Could you check a few things on this model? Use its own coordinates, in mm. Coordinates: 2 decimals unless noted, no trailing zeros. Loops run counter-clockwise (first coordinate to the right, second up) from the corner with the lowest first, then second, coordinate; pieces in that order, holes last. Notation, with made-up numbers: M 37,86 L 44,86 A25 cw 44,112 Z; hole C 11.25,-3 d3. An arc over 180 degrees is marked long. Write each question's results on one line, items separated by ' | '.
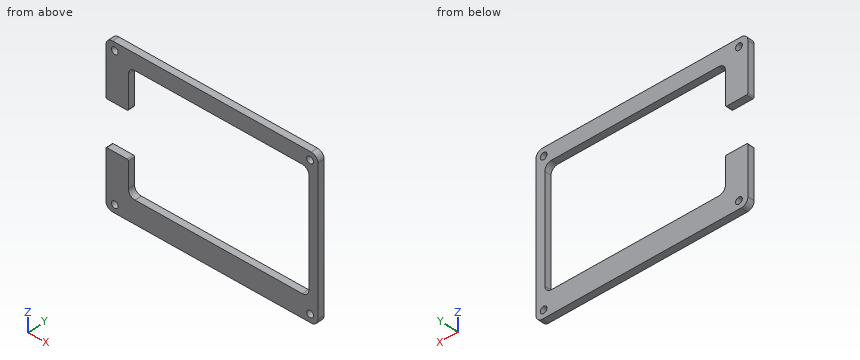
```python
from build123d import *

# Parameters (mm, degrees)
SKETCH1_W           = 94.5
SKETCH1_H           = 70
BOSS_EXTRUDE1_DEPTH = 3
SKETCH3_R           = 1.5
CUT_EXTRUDE2_DEPTH  = 59.877521177
FILLET2_R           = 3
SKETCH5_W           = 10
SKETCH5_H           = 20
CUT_EXTRUDE3_DEPTH  = 59.877521177
FILLET3_R           = 3
FILLET4_R           = 0.5


with BuildPart() as part:
    # Sketch1 → Boss-Extrude1 (new body)
    with BuildSketch(Plane(origin=(0, 0, 0), x_dir=(1, 0, 0), z_dir=(0, 1, 0))):
        Rectangle(SKETCH1_W, SKETCH1_H)
    extrude(amount=BOSS_EXTRUDE1_DEPTH)

    # Sketch3 → Cut-Extrude2 (cut, through all)
    with BuildSketch(Plane(origin=(0, 3, 0), x_dir=(1, 0, 0), z_dir=(0, 1, 0))):
        with Locations(Location((43.75, 31.5, 0), (0, 0, 270))):
            Circle(SKETCH3_R)
        with Locations(Location((-43.25, 31.5, 0), (0, 0, 270))):
            Circle(SKETCH3_R)
        with Locations(Location((-43.25, -31.5, 0), (0, 0, 270))):
            Circle(SKETCH3_R)
        with Locations(Location((43.75, -31.5, 0), (0, 0, 270))):
            Circle(SKETCH3_R)
    extrude(amount=-CUT_EXTRUDE2_DEPTH, mode=Mode.SUBTRACT)

    # Fillet2
    fillet2_edges = [part.edges().sort_by_distance(p)[0] for p in [
        (47.25, 1.5, 35),
        (-47.25, 1.5, 35),
        (-47.25, 1.5, -35),
        (47.25, 1.5, -35),
    ]]
    fillet(fillet2_edges, radius=FILLET2_R)

    # Sketch5 → Cut-Extrude3 (cut, through all)
    with BuildSketch(Plane(origin=(0, 3, 0), x_dir=(1, 0, 0), z_dir=(0, 1, 0))):
        Polygon((-30, -28), (-37.25, -28), (-37.25, 25), (43.25, 25), (43.25, -28), align=None)
        with Locations((-42.25, 0)):
            Rectangle(SKETCH5_W, SKETCH5_H)
    extrude(amount=-CUT_EXTRUDE3_DEPTH, mode=Mode.SUBTRACT)

    # Fillet3
    fillet3_edges = [part.edges().sort_by_distance(p)[0] for p in [
        (43.25, 1.5, 28),
        (-37.25, 1.5, 28),
        (-37.25, 1.5, -25),
        (43.25, 1.5, -25),
    ]]
    fillet(fillet3_edges, radius=FILLET3_R)

    # Fillet4
    fillet4_edges = [part.edges().sort_by_distance(p)[0] for p in [
        (-37.25, 1.5, 10),
        (-47.25, 1.5, 10),
        (-47.25, 1.5, -10),
        (-37.25, 1.5, -10),
    ]]
    fillet(fillet4_edges, radius=FILLET4_R)


solid = part.part
```
(1) Imagine slicing it at A-A, the plane x = -11. List the corners of the cut face in (y, z) for me.
Reported:
outline: M 0,-35 L 3,-35 L 3,-25 L 0,-25 Z; M 0,28 L 3,28 L 3,35 L 0,35 Z
(2) Imagine slicing it at C-C, the plane y = 0.8. List the corners of the cut face in (x, z) for me, and give its area (3 significant figures).
Reported:
outline: M -47.25,-32 A3 ccw -44.25,-35 L 44.25,-35 A3 ccw 47.25,-32 L 47.25,32 A3 ccw 44.25,35 L -44.25,35 A3 ccw -47.25,32 L -47.25,10.5 A0.5 ccw -46.75,10 L -37.75,10 A0.5 ccw -37.25,10.5 L -37.25,25 A3 cw -34.25,28 L 40.25,28 A3 cw 43.25,25 L 43.25,-22 A3 cw 40.25,-25 L -34.25,-25 A3 cw -37.25,-22 L -37.25,-10.5 A0.5 ccw -37.75,-10 L -46.75,-10 A0.5 ccw -47.25,-10.5 Z; hole C -43.25,-31.5 d3; hole C -43.25,31.5 d3; hole C 43.75,-31.5 d3; hole C 43.75,31.5 d3 | area: 2,120 mm2
(3) Will these pins go through, and if not, where does the flat tip stop? P1, Ø4, axis at x = 43.75, z = 31.5, coming from the +Y side; P2, Ø3, axis at x = 9, z = -22, coming from the -Y side.
Reported:
P1: stops at y = 3 | P2: passes through
(4) Please list where these lines run through material, in increasing order: probe 1 along X at (y, z) = (1.35, 31.5); probe 2 along Z at (x, y) = (-15, 1.4); probe 3 along X at (y, z) = (2.2, 14.5). Write a range as from..to.
Reported:
probe 1: x = -47.25..-44.75, -41.75..42.25, 45.25..47.25 | probe 2: z = -35..-25, 28..35 | probe 3: x = -47.25..-37.25, 43.25..47.25
(5) Imagine slicing it at B-B, the plane z = 12. List the corners of the cut face in (x, y) for me, and give its area (3 significant figures).
Reported:
outline: M -47.25,0 L -37.25,0 L -37.25,3 L -47.25,3 Z; M 43.25,0 L 47.25,0 L 47.25,3 L 43.25,3 Z | area: 42.0 mm2
